Could you check a few things on this drawing? It's one solid part, dimensions in mm from its lowest x, y, z. Give positions to 0.01 mm unless a question says otherwise; leave off trailing zeros. Loops run counter-clockwise (first coordinate to the right, second up) from the corner with the lowest first, then second, coordinate; pieces in that order, holes last. Notation, with made-up numbers: (-35.75, 56.25) - (-15.75, 56.25) arc R33 ccw to (-15.75, 92.25) - close; hole circle Ø3 at (-23.5, 45). An arc over 180 degrees is marked (long way). Return JSON: item names as keys, results as strings. Group by question number.
(1) If we section it at B-B (x = 50): Please give me the cut outline in (y, z).
(2) If we section it at D-D (x = 184): Please give me the cut outline in (y, z), then the cut area to 3 significant figures.
(3) I need wall thicknesses on probe 1 along Y at (x, z) = (50, 3); probe 2 along Y at (x, z) = (174, 8.5); probe 3 along X at (y, z) = (58, 2). Which ranges of each line are inside material? Lowest first, please. Write a range as [from, to].
(4) If we section it at C-C (z = 3.5): Please give me the cut outline in (x, y), then the cut area to 3 significant figures.
(5) For P1, Ø5, axis at x = 156, z = 3, coming from the +Y side; P2, Ø5, axis at x = 173, z = 7, coming from the -Y side; P3, Ø3, axis at y = 96, z = 4.5, coming from the +X side, each with a flat end and sliding along its axis, tell me the tip position at first contact or that it passes through.
(6) If we section it at A-A (y = 50): Please give me the cut outline in (x, z), then the cut area to 3 significant figures.
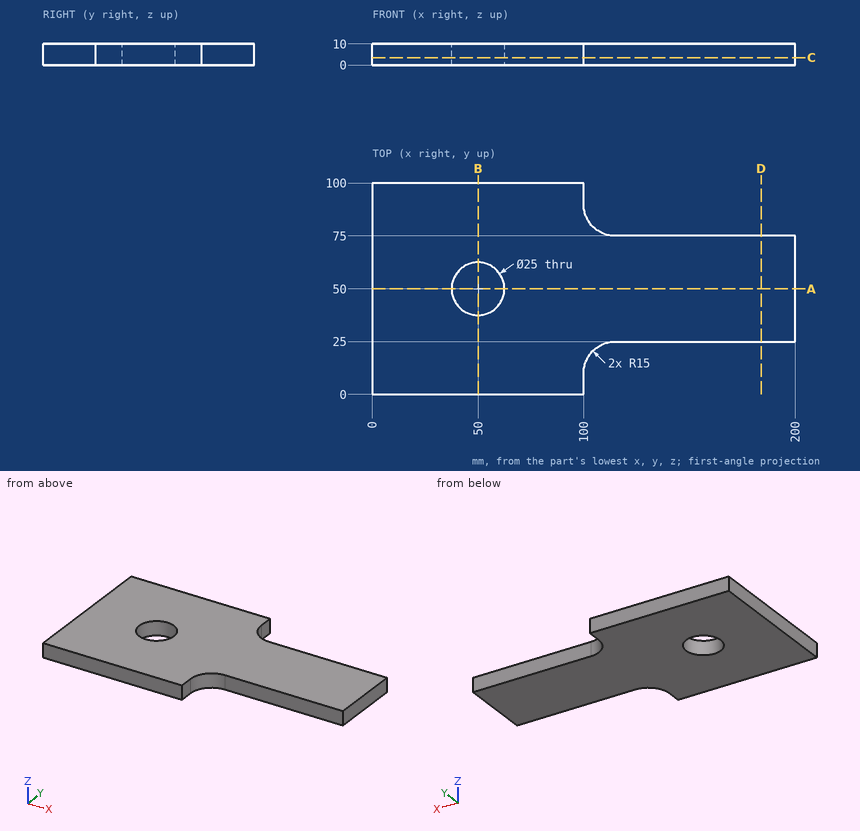
Values:
{
 "1": {"outline": "(0, 0) - (37.5, 0) - (37.5, 10) - (0, 10) - close; (62.5, 0) - (100, 0) - (100, 10) - (62.5, 10) - close"},
 "2": {"outline": "(25, 0) - (75, 0) - (75, 10) - (25, 10) - close", "area": "500 mm2"},
 "3": {"probe 1": "[0, 37.5], [62.5, 100]", "probe 2": "[25, 75]", "probe 3": "[0, 40.4], [59.6, 200]"},
 "4": {"outline": "(0, 0) - (100, 0) - (100, 10) arc R15 cw to (115, 25) - (200, 25) - (200, 75) - (115, 75) arc R15 cw to (100, 90) - (100, 100) - (0, 100) - close; hole circle Ø25 at (50, 50)", "area": "14,600 mm2"},
 "5": {"P1": "y = 75", "P2": "y = 25", "P3": "x = 100"},
 "6": {"outline": "(0, 0) - (37.5, 0) - (37.5, 10) - (0, 10) - close; (62.5, 0) - (200, 0) - (200, 10) - (62.5, 10) - close", "area": "1,750 mm2"}
}
